For this review, take the finished solid that the model builds, in its own axes (mm). A direction names the side the tool comes from. Give positions to 0.01 mm unless a question says otherwise; leave off trailing zeros. Loops run counter-clockwise (first coordinate to the right, second up) from the corner with the lowest first, then second, coordinate; pieces in that order, holes last. Notation, with made-up numbers: (80.5, -30) - (129.5, -30) arc R17 cw to (129.5, -8) - close; hole circle Ø4 at (2.5, -3). An arc over 180 degrees is marked (long way). Answer in a Markdown table with one row per item.
```python
from build123d import *

# Parameters (mm, degrees)
F_01_EIGHT_MILLIMETRE_TRACK_BLANK_DEPTH        = 8
F_02_LOWER_CAGE_TIE_LANDING_DEPTH              = 8
F_03_BUMP_END_SUPPORT_LANDING_DEPTH            = 8
F_04_START                                     = -0.1
S04_RELIEF_FOR_THE_SWEPT_FLOATING_GUID_R       = 45.5
F_04_RELIEF_FOR_THE_SWEPT_FLOATING_GUIDE_DEPTH = 8.2
F_05_START                                     = -0.1
F_05_CONCENTRIC_GUIDE_AND_TANGENT_STOP_F_DEPTH = 8.2
F_06_START                                     = -0.1
S06_SUPPORT_FASTENERS_R                        = 3.3
F_06_SUPPORT_FASTENERS_DEPTH                   = 8.2
F_07_START                                     = -0.1
S07_BUMP_END_SUPPORT_REGISTER_UNDERSID_R       = 5.06
F_07_BUMP_END_SUPPORT_REGISTER_UNDERSIDE_DEPTH = 1.35
F_08_START                                     = 4.5
S08_FLUSH_BUTTON_SCREW_COUNTERBORE_OUT_R       = 5.5
F_08_FLUSH_BUTTON_SCREW_COUNTERBORE_OUTB_DEPTH = 3.6
F_01_START                                     = -0.1
S01_FULL_DIAMETER_LOCATING_SEAT_FOR_PR_R       = 8.15
F_01_FULL_DIAMETER_LOCATING_SEAT_FOR_PRI_DEPTH = 1.35


with BuildPart() as part:
    # S01 - Eight millimetre track blank → 01 - Eight millimetre track blank (new body)
    with BuildSketch(Plane.XY):
        with BuildLine():
            Line((25.527156043, -37.845565187), (42.69437818, -63.297018665))
            ThreePointArc((42.69437818, -63.297018665), (74.240443422, -17.82355353), (66.77721464, 37.015214506))
            Line((66.77721464, 37.015214506), (39.926389631, 22.131559164))
            ThreePointArc((39.926389631, 22.131559164), (44.388686866, -10.65678086), (25.527156043, -37.845565187))
        make_face()
    extrude(amount=F_01_EIGHT_MILLIMETRE_TRACK_BLANK_DEPTH)

    # S02 - Lower cage tie landing → 02 - Lower cage tie landing (add)
    with BuildSketch(Plane.XY):
        with BuildLine():
            Line((-1.286113116, -44.083049206), (34.568787274, -39.433085863))
            ThreePointArc((34.568787274, -39.433085863), (45.771851184, -48.063923541), (37.141013506, -59.266987451))
            Line((37.141013506, -59.266987451), (1.286113116, -63.916950794))
            ThreePointArc((1.286113116, -63.916950794), (-9.916950794, -55.286113116), (-1.286113116, -44.083049206))
        make_face()
    extrude(amount=F_02_LOWER_CAGE_TIE_LANDING_DEPTH)

    # S03 - Bump end support landing → 03 - Bump end support landing (add)
    with BuildSketch(Plane.XY):
        with BuildLine():
            Line((45.572351488, 20.615526776), (42.574781821, 26.253135379))
            ThreePointArc((42.574781821, 26.253135379), (47.123018152, 41.129746091), (61.999628864, 36.58150976))
            Line((61.999628864, 36.58150976), (64.997198531, 30.943901157))
            ThreePointArc((64.997198531, 30.943901157), (60.4489622, 16.067290445), (45.572351488, 20.615526776))
        make_face()
    extrude(amount=F_03_BUMP_END_SUPPORT_LANDING_DEPTH)

    # S04 - Relief for the swept floating guide barrels → 04 - Relief for the swept floating guide barrels (cut)
    with BuildSketch(Plane.XY.offset(F_04_START)):
        Circle(S04_RELIEF_FOR_THE_SWEPT_FLOATING_GUID_R)
    extrude(amount=F_04_RELIEF_FOR_THE_SWEPT_FLOATING_GUIDE_DEPTH, mode=Mode.SUBTRACT)

    # S05 - Concentric guide and tangent stop faces → 05 - Concentric guide and tangent stop faces (cut)
    with BuildSketch(Plane.XY.offset(F_05_START)):
        with BuildLine():
            Line((34.862224899, -39.454375867), (45.92013859, -51.968869257))
            ThreePointArc((45.92013859, -51.968869257), (66.319734826, -20.275977723), (67.130143118, 17.405929591))
            Line((67.130143118, 17.405929591), (50.9647013, 13.214451233))
            ThreePointArc((50.9647013, 13.214451233), (50.349445401, -15.393370254), (34.862224899, -39.454375867))
        make_face()
    extrude(amount=F_05_CONCENTRIC_GUIDE_AND_TANGENT_STOP_F_DEPTH, mode=Mode.SUBTRACT)

    # S06 - Support fasteners → 06 - Support fasteners (cut)
    with BuildSketch(Plane.XY.offset(F_06_START)):
        with Locations(Location((0, -54, 0), (0, 0, 180))):
            Circle(S06_SUPPORT_FASTENERS_R)
        with Locations(Location((52.287205343, 31.41732257, 0), (0, 0, 180))):
            Circle(S06_SUPPORT_FASTENERS_R)
    extrude(amount=F_06_SUPPORT_FASTENERS_DEPTH, mode=Mode.SUBTRACT)

    # S07 - Bump end support register underside → 07 - Bump end support register underside (cut)
    with BuildSketch(Plane.XY.offset(F_07_START)):
        with Locations(Location((52.287205343, 31.41732257, 0), (0, 0, 180))):
            Circle(S07_BUMP_END_SUPPORT_REGISTER_UNDERSID_R)
    extrude(amount=F_07_BUMP_END_SUPPORT_REGISTER_UNDERSIDE_DEPTH, mode=Mode.SUBTRACT)

    # S08 - Flush button screw counterbore outboard → 08 - Flush button screw counterbore outboard (cut)
    with BuildSketch(Plane.XY.offset(F_08_START)):
        with Locations(Location((52.287205343, 31.41732257, 0), (0, 0, 180))):
            Circle(S08_FLUSH_BUTTON_SCREW_COUNTERBORE_OUT_R)
    extrude(amount=F_08_FLUSH_BUTTON_SCREW_COUNTERBORE_OUTB_DEPTH, mode=Mode.SUBTRACT)

    # S01 - Full diameter locating seat for printed post → 01 - Full diameter locating seat for printed post (cut)
    with BuildSketch(Plane.XY.offset(F_01_START)):
        with Locations(Location((52.287205346, 31.41732257, 0), (0, 0, 180))):
            Circle(S01_FULL_DIAMETER_LOCATING_SEAT_FOR_PR_R)
    extrude(amount=F_01_FULL_DIAMETER_LOCATING_SEAT_FOR_PRI_DEPTH, mode=Mode.SUBTRACT)


solid = part.part
```
1. Clearance check with flat-ended pins moving along their axes: pin 1 (3 mm diameter, centred on y = 8.5, z = 7, fed in from +X); pin 2 (1 mm diameter, centred on y = 14.5, z = 5.5, fed in from -X); pin 3 (4 mm diameter, centred on x = 61.5, z = 2.5, fed in from +Y). State where each tip first meets the part, or that it passes through.
Values:
| item | result |
|---|---|
| pin 1 | stops at x = 76.03 |
| pin 2 | stops at x = 43.12 |
| pin 3 | stops at y = 39.72 |
2. We need section D-D, the plane x = 32.5. Give the boundary of the cut face in (y, z).
Values:
| item | result |
|---|---|
| outline | (-59.87, 0) - (-32.06, 0) - (-32.06, 8) - (-59.87, 8) - close |
3. Wall thickness on line 1 (X direction, y = -0.5, z = 7); line 2 (Z direction, x = 49, y = 33); line 3 (X direction, y = 29.5, z = 0.5): over which ranges is each line inside the solid? List them lowest first. Write a range as [from, to].
Values:
| item | result |
|---|---|
| line 1 | x = [45.65, 52.65], [69.35, 76.35] |
| line 2 | z = [1.25, 4.5] |
| line 3 | x = [41.46, 44.37], [60.21, 70.42] |
4. We need section B-B, the plane y = -54. Give the boundary of the cut face in (x, z).
Values:
| item | result |
|---|---|
| outline | (-10, 0) - (-3.3, 0) - (-3.3, 8) - (-10, 8) - close; (3.3, 0) - (53.98, 0) - (53.98, 8) - (3.3, 8) - close |
5. For faces 1 (the face through (52, 35, 4.5)), 2 (the face through (59.16, 15.34, 3.94)), 3 (the face through (64.87, 35.96, 3.94)), list the 3-axis set-ups (+Z, -Z, +X, -X, +Y, -Y) from which the entire face can be reached by the end or side of a thin tool; tool diameter is ignored.
Values:
| item | result |
|---|---|
| face 1 | +Z |
| face 2 | +Z, -Z |
| face 3 | +Z, -Z, +Y |
6. Mouldability with a two-part tool opening along Y and no side actions: class faces 4 (the face through (43, -22, 0)), 5 (the face through (53.479, 36.787, 6.226)), 6 (the face through (26.371, -39.097, 3.944)), 7 (the face through (38.384, -59.025, 3.944)) as released by +Y, released by -Y, zero draft, split by the parting line, or undercut.
Values:
| item | result |
|---|---|
| face 4 | zero draft |
| face 5 | undercut |
| face 6 | undercut |
| face 7 | released by -Y |
7. We need section A-A, the plane x = 0. Give the boundary of the cut face in (y, z).
Values:
| item | result |
|---|---|
| outline | (-64, 0) - (-57.3, 0) - (-57.3, 8) - (-64, 8) - close; (-50.7, 0) - (-45.5, 0) - (-45.5, 8) - (-50.7, 8) - close |
8. We need section C-C, the plane z = 5.75. Give the boundary of the cut face in (x, y).
Values:
| item | result |
|---|---|
| outline | (-4.83, -45.24) arc R10 ccw to (1.29, -63.92) - (37.14, -59.27) arc R10 ccw to (39.55, -58.64) - (42.69, -63.3) arc R76.35 ccw to (66.78, 37.02) - (62.91, 34.87) - (62, 36.58) arc R11 ccw to (42.57, 26.25) - (43.66, 24.2) - (39.93, 22.13) arc R45.65 cw to (25.53, -37.85) - (27.24, -40.38) - (18.66, -41.5) arc R45.5 cw to start; hole circle Ø6.6 at (0, -54); hole (34.86, -39.45) - (45.92, -51.97) arc R69.35 ccw to (67.13, 17.41) - (50.96, 13.21) arc R52.65 cw to start; hole circle Ø11 at (52.29, 31.42) |
